Could you check a few things on this drawing? It's one solid part, dimensions in mm from its lowest x, y, z. Round coordinates to 2 decimals unless told otherwise and drop trailing zeros. Write each loop counter-clockwise with the first axis right and the second up, starting at its lowest first coordinate (ties: lowest second). Pieces come first, ordered by that corner, then holes. Notation, with made-up numbers: (39.5, 0) - (52.5, 0) arc R16 ccw to (52.5, 25) - close; hole circle Ø6 at (72, 74.5). An arc over 180 degrees is marked (long way). Write item = value, one per line. Start each with the question number.
Item 1: If I drill on line 1 along Y through (x, z) = (7.21, 1.3) (1 decimal); line 2 along X through (y, z) = (8, 2.2) (1 decimal); line 3 along Y through (x, z) = (60, 1.8) (1 decimal), over which ranges is the centre line in solid material (lowest first)? Write a range as [from, to].
Item 2: For P1, Ø1.5, axis at y = 27, z = 1.5, coming from the +X side (1 decimal); P2, Ø1.5, axis at y = 23.5, z = 2, coming from the +X side (1 decimal), each with a flat end and sliding along its axis, tell me the tip position at first contact or that it passes through.
Item 3: If we section it at A-A (x = 7.21): Please give me the cut outline in (y, z) (1 decimal).
Item 4: If we section it at C-C (z = 1.8): Give the number of separate pieces and of enclosed holes in the cut face.
Item 5: If we section it at D-D (x = 15.5): Please give me the cut outline in (y, z) (1 decimal).
Item 6: Thinking about a two-plate mould opening in Y: for the marked faces 1, 2 and 3, which applies, pulls with the +Y half, pulls with the -Y half, needs draft (parallel to the pull), parting line crosses it, or undercut?
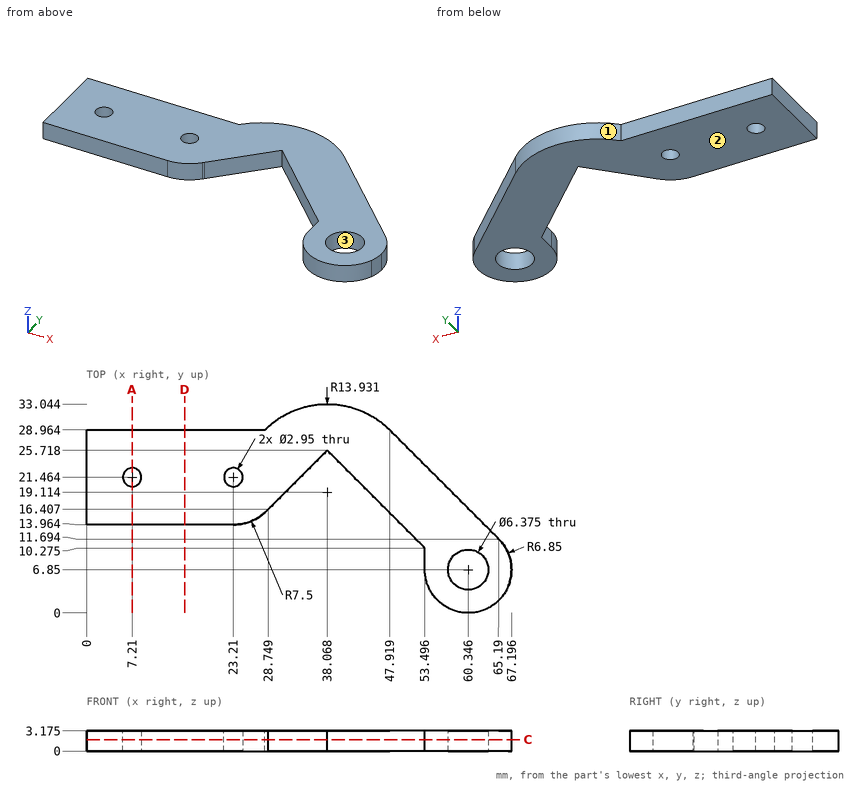
Reply:
q1.line_1 = [14, 20], [22.9, 29]
q1.line_2 = [53.5, 57.4], [63.3, 67.1]
q1.line_3 = [0, 3.7], [10, 16.9]
q2.P1 = 50.6
q2.P2 = 54.1
q3.outline = (14, 0) - (20, 0) - (20, 3.2) - (14, 3.2) - close; (22.9, 0) - (29, 0) - (29, 3.2) - (22.9, 3.2) - close
q4.separate_pieces = 1
q4.enclosed_holes = 3
q5.outline = (14, 0) - (29, 0) - (29, 3.2) - (14, 3.2) - close
q6.face_1 = pulls with the +Y half
q6.face_2 = needs draft
q6.face_3 = undercut
